from build123d import *

# Parameters (mm, degrees)
F0_W     = 33.75
F0_H     = 16.5
F1_DEPTH = 8.25
F2_R     = 4
F3_R     = 2


with BuildPart() as f1:
    # F0 (on Top) → F1 (new body)
    with BuildSketch(Plane.XY):
        Rectangle(F0_W, F0_H)
    extrude(amount=F1_DEPTH)

    # F2
    f2_edges = [f1.edges().sort_by_distance(p)[0] for p in [
        (-16.875, 0, 8.25),
        (-16.875, 0, 0),
    ]]
    fillet(f2_edges, radius=F2_R)

    # F3
    f3_edges = [f1.edges().sort_by_distance(p)[0] for p in [
        (2, -8.25, 8.25),
        (2, 8.25, 8.25),
        (16.875, 0, 8.25),
        (16.875, 0, 0),
        (16.875, -8.25, 4.125),
        (16.875, 8.25, 4.125),
    ]]
    fillet(f3_edges, radius=F3_R)


solid = f1.part
The model under review builds one solid part; all positions refer to its coordinate system, in mm. Give positions to 0.01 mm unless a question says otherwise; leave off trailing zeros. Write each loop counter-clockwise with the first axis right and the second up, starting at its lowest first coordinate (ties: lowest second). Pieces come first, ordered by that corner, then holes. Notation, with made-up numbers: M 0.5,-34 L 44.5,-34 A29 cw 44.5,-5 Z; hole C 68.5,-3.5 d10. An arc over 180 degrees is marked long. One line per question, with ' | ' between items. Start each with the question number.
Item 1: We need section B-B on x = 5. Write out the cut boundary in (y, z), plus the area to 3 significant figures.
Item 2: We need section A-A on y = -0.25. Write out the cut boundary in (x, z) (3 decimals).
Item 3: Wall thickness on line 1 (Z direction, x = 15, y = -1.5); line 2 (X direction, y = -2.25, z = 3.5) (3 decimals); line 3 (Z direction, x = 12.5, y = 7.5): over which ranges is each line inside the solid? List them lowest first. Write a range as from..to.
Results found:
1) outline: M -8.25,2 A2 ccw -6.25,0 L 6.25,0 A2 ccw 8.25,2 L 8.25,6.25 A2 ccw 6.25,8.25 L -6.25,8.25 A2 ccw -8.25,6.25 Z | area: 133 mm2
2) outline: M -16.875,4 A4 ccw -12.875,0 L 14.875,0 A2 ccw 16.875,2 L 16.875,6.25 A2 ccw 14.875,8.25 L -12.875,8.25 A4 ccw -16.875,4.25 Z
3) line 1: z = 0..8.25 | line 2: x = -16.844..16.875 | line 3: z = 0.44..7.81
